Read the model definition and answer for the solid it produces. Units are mm, in the model's axes. A direction names the side the tool comes from. Round coordinates to 2 decimals unless told otherwise and drop trailing zeros. Loops run counter-clockwise (first coordinate to the right, second up) from the corner with the lowest first, then second, coordinate; pieces in that order, holes last. Notation, with made-up numbers: (76, -19) - (116, -19) arc R29 cw to (116, 16) - close; hole circle Ø3 at (-3.75, 50.25). An arc over 180 degrees is marked (long way). Use one line per item in the form item = value. Start each with the question number.
```python
from build123d import *

# Parameters (mm, degrees)
SKETCH_1_W             = 500
SKETCH_1_H             = 440
EXTRUDE_1_DEPTH        = 520
SKETCH_2_W             = 520
SKETCH_2_H             = 450
EXTRUDE_2_DEPTH        = 30
SKETCH_3_W             = 420
SKETCH_3_H             = 160
EXTRUDE_3_DEPTH        = 5
SKETCH_4_W             = 80
SKETCH_4_H             = 30.476190476
CUT_EXTRUDE_2_DEPTH    = 10
PATTERN_LINEAR_1_COUNT = 2
PATTERN_LINEAR_1_PITCH = 190


with BuildPart() as part:
    # 草图1 → 凸台-拉伸1 (new body)
    with BuildSketch(Plane(origin=(0, 0, 0), x_dir=(1, 0, 0), z_dir=(0, 1, 0))):
        Rectangle(SKETCH_1_W, SKETCH_1_H)
    extrude(amount=EXTRUDE_1_DEPTH)

    # 草图2 → 凸台-拉伸2 (add)
    with BuildSketch(Plane(origin=(0, 520, 0), x_dir=(1, 0, 0), z_dir=(0, 1, 0))):
        with Locations((0, -5)):
            Rectangle(SKETCH_2_W, SKETCH_2_H)
    extrude(amount=-EXTRUDE_2_DEPTH)

    # 草图3 → 凸台-拉伸3 (add)
    with BuildSketch(Plane.XY.offset(220)):
        with Locations((0, 380)):
            Rectangle(SKETCH_3_W, SKETCH_3_H)
    extrude_3 = extrude(amount=EXTRUDE_3_DEPTH)

    # 草图4 → 切除-拉伸2 (cut)
    with BuildSketch(Plane.XY.offset(225)):
        with Locations((0, 380)):
            Rectangle(SKETCH_4_W, SKETCH_4_H)
    cut_extrude_2 = extrude(amount=-CUT_EXTRUDE_2_DEPTH, mode=Mode.SUBTRACT)

    # 阵列(线性)1: 凸台-拉伸3, 切除-拉伸2 ×2
    with Locations(*[(0, -i * PATTERN_LINEAR_1_PITCH, 0) for i in range(1, PATTERN_LINEAR_1_COUNT)]):
        add(extrude_3)
        add(cut_extrude_2, mode=Mode.SUBTRACT)


solid = part.part
```
1) A cutting plane is placed at A-A on y = 332.5. Write down the section's boundary in (x, z).
2) Straight lines are drawn through the part: line 1 (X direction, y = 479.5, z = -49.5); line 2 (Z direction, x = 203, y = 139.5); line 3 (Z direction, x = -49.5, y = 72). For each, find the intervals that lie inside material, in ascending order. Write a range as from..to.
3) For faces 1 (the flat face through (250, 242, 3)), 2 (the flat face through (-3, 399, 225)), 3 (the flat face through (-250, 242, 3)), 4 (the flat face through (-1, 380, 215)), determine the directions among +Z, -Z, +X, -X, +Y, -Y from which every point of the face is accessible in a straight line to the end or side of a thin tool.
4) A cutting plane is placed at C-C on x = -19.5. Write down the section's boundary in (y, z), plus the area to 3 significant figures.
5) A cutting plane is placed at D-D on y = 94.5. Write down the section's boundary in (x, z).
6) A cutting plane is placed at B-B on z = -44. Write down the section's boundary in (x, y).
7) Flat-ended cylindrical pins translate along their axes: pin 1 (5.5 mm diameter, centred on y = 215, z = 222, fed in from +X); pin 2 (8 mm diameter, centred on y = 116, z = 150.5, fed in from -X); pin 3 (11 mm diameter, centred on x = -14, z = 222.5, fed in from -Y); pin 4 (4 mm diameter, centred on y = 208, z = 223.5, fed in from -X). Find the tip coordinate at first contact, or state that the pin passes through.
8) Determine the mould class of faces 5 (the flat face through (-1, 190, 215)), 6 (the flat face through (-4, 264, -220)), 7 (the flat face through (260, 505, 8)), 8 (the flat face through (-260, 505, 8)) for opening direction X: +X half, -X half, draft (parallel to the pull), parting line (faces both ways), or undercut.
Checks:
q1.outline = (-250, -220) - (250, -220) - (250, 220) - (210, 220) - (210, 225) - (-210, 225) - (-210, 220) - (-250, 220) - close
q2.line_1 = -250..250
q2.line_2 = -220..225
q2.line_3 = -220..220
q3.face_1 = +Z, -Z, +X, -Y
q3.face_2 = +Z, +X, -X, -Y
q3.face_3 = +Z, -Z, -X, -Y
q3.face_4 = +Z
q4.outline = (0, -220) - (520, -220) - (520, 230) - (490, 230) - (490, 220) - (460, 220) - (460, 225) - (395.24, 225) - (395.24, 215) - (364.76, 215) - (364.76, 225) - (300, 225) - (300, 220) - (270, 220) - (270, 225) - (205.24, 225) - (205.24, 215) - (174.76, 215) - (174.76, 225) - (110, 225) - (110, 220) - (0, 220) - close
q4.area = 230,000 mm²
q5.outline = (-250, -220) - (250, -220) - (250, 220) - (-250, 220) - close
q6.outline = (-260, 490) - (-250, 490) - (-250, 0) - (250, 0) - (250, 490) - (260, 490) - (260, 520) - (-260, 520) - close
q7.pin_1 = 250
q7.pin_2 = -250
q7.pin_3 = 0
q7.pin_4 = -210
q8.face_5 = undercut
q8.face_6 = draft
q8.face_7 = +X half
q8.face_8 = -X half
